Study the drawing (mm; zero at the part's minimum x, y, z) and answer. A direction names the side the tool comes from. Give positions to 0.01 mm unless a question says otherwise; leave off trailing zeros. Order: outer loops, then holes, each group sorted by start corner. A loop starts at its lowest first (then second) coordinate and runs counter-clockwise, first axis right, second up.
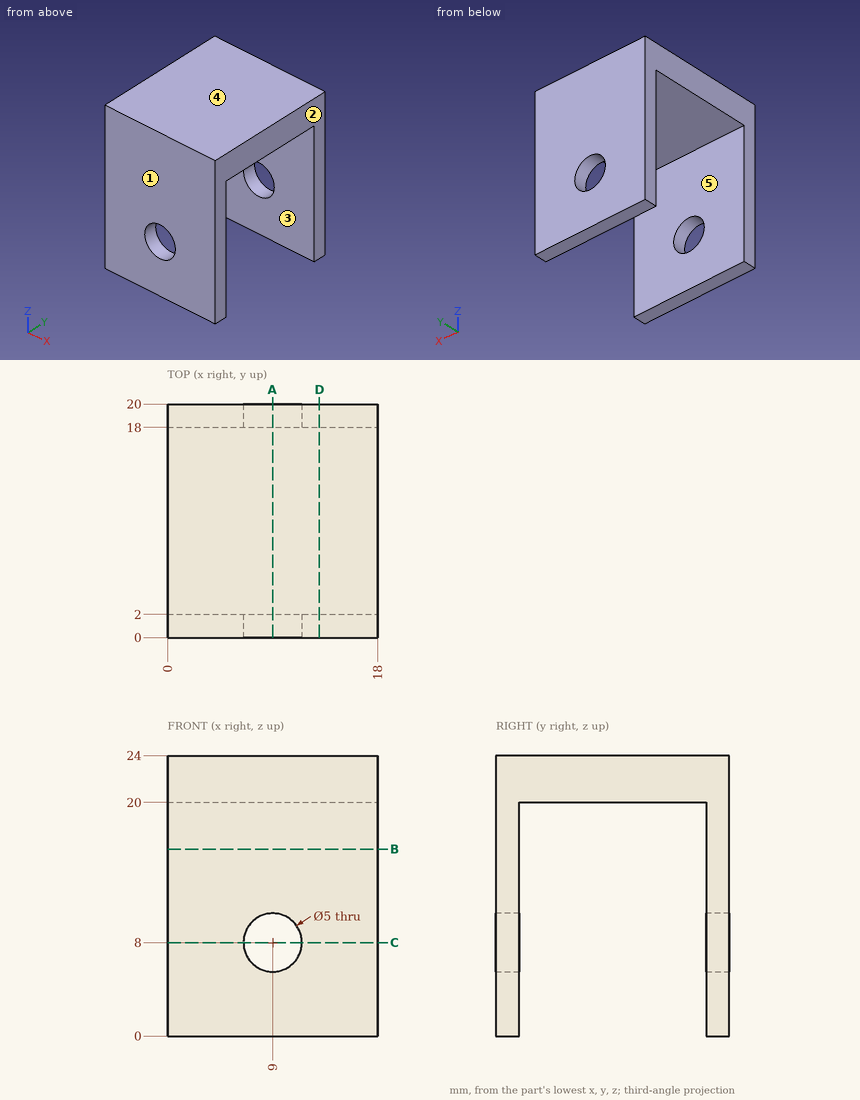
1) Find section B-B (z = 16). Write down the section's boundary in (x, y), then the cut area to 3 significant figures.
Geometry says:
outline: (0, 0) - (18, 0) - (18, 2) - (0, 2) - close; (0, 18) - (18, 18) - (18, 20) - (0, 20) - close
area: 72.0 mm2
2) Find section C-C (z = 8). Write down the section's boundary in (x, y), then the cut area to 3 significant figures.
Geometry says:
outline: (0, 0) - (6.5, 0) - (6.5, 2) - (0, 2) - close; (0, 18) - (6.5, 18) - (6.5, 20) - (0, 20) - close; (11.5, 0) - (18, 0) - (18, 2) - (11.5, 2) - close; (11.5, 18) - (18, 18) - (18, 20) - (11.5, 20) - close
area: 52.0 mm2
3) Find section A-A (x = 9). Write down the section's boundary in (y, z), then the cut area to 3 significant figures.
Geometry says:
outline: (0, 0) - (2, 0) - (2, 5.5) - (0, 5.5) - close; (0, 10.5) - (2, 10.5) - (2, 20) - (18, 20) - (18, 10.5) - (20, 10.5) - (20, 24) - (0, 24) - close; (18, 0) - (20, 0) - (20, 5.5) - (18, 5.5) - close
area: 140 mm2
4) Find section D-D (x = 13). Write down the section's boundary in (y, z), then the cut area to 3 significant figures.
Geometry says:
outline: (0, 0) - (2, 0) - (2, 20) - (18, 20) - (18, 0) - (20, 0) - (20, 24) - (0, 24) - close
area: 160 mm2
5) Straight lines are drawn through the part: probe 1 along X at (y, z) = (1.1, 8); probe 2 along Y at (x, z) = (8, 12.25); probe 3 along Z at (x, y) = (17, 8.75). For each, find the intervals that lie inside material, in ascending order.
Geometry says:
probe 1: x = 0 to 6.5, 11.5 to 18
probe 2: y = 0 to 2, 18 to 20
probe 3: z = 20 to 24
6) A tool of negligible diameter and unlimited length cuts with its end or side. For the marked faces 4 and 5, from which of +Z, -Z, +X, -X, +Y, -Y can it reach the whole face along a straight path? Write none if from no direction.
Geometry says:
face 4: +Z, +X, -X, +Y, -Y
face 5: -Z, +X, -X
7) For a pull along Y with two mould halves and no side action, classify the marked faces 1, 2 and 3 as +Y half, -Y half, draft (parallel to the pull), parting line (faces both ways), or undercut.
Geometry says:
face 1: -Y half
face 2: draft
face 3: undercut
8) Given P1, Ø4.5, axis at x = 9, z = 8, coming from the +Y side; P2, Ø6.5, axis at x = 9, z = 8, coming from the -Y side; P3, Ø5, axis at x = 12.5, y = 12.5, coming from the -Z side, each flat-ended and moving along its own axis, determine where each tip first touches the part or whether it passes through.
Geometry says:
P1: passes through
P2: stops at y = 0
P3: stops at z = 20
